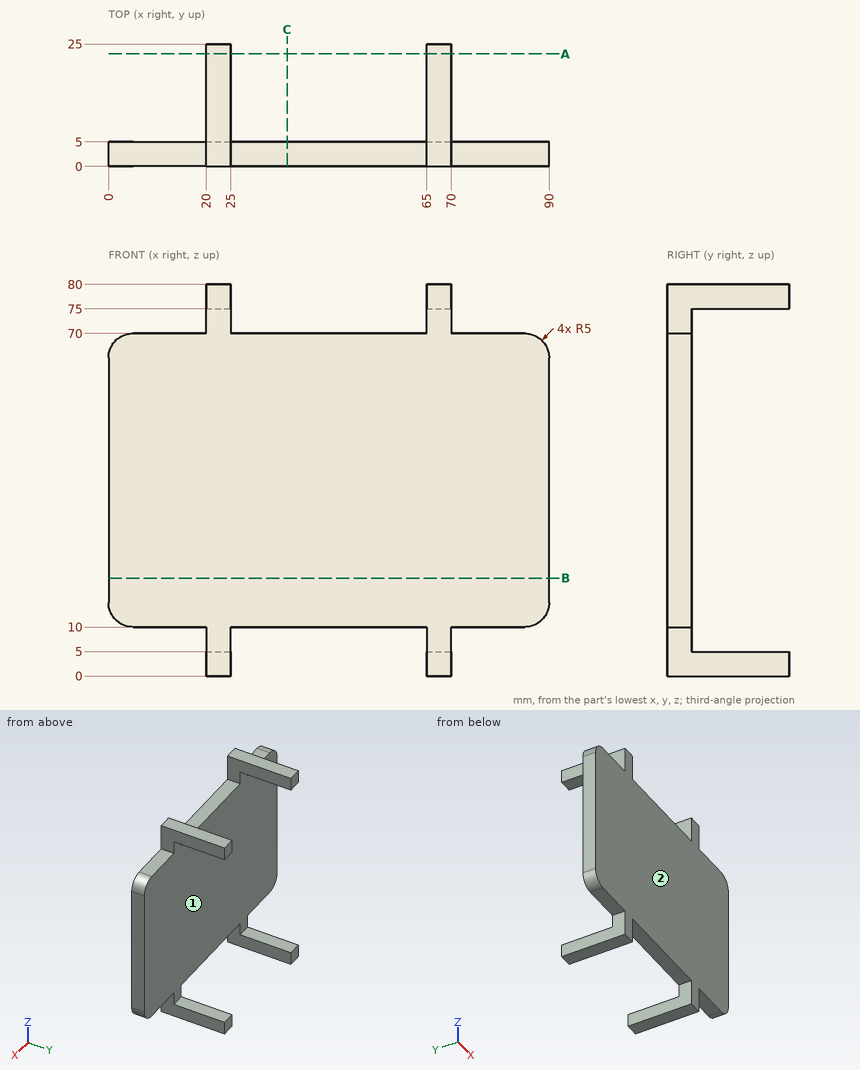
For this review, use the dimensioned drawing (mm, ordinates from the lowest corner) and the shaded views. A direction names the side the tool comes from. Round coordinates to 2 decimals unless told otherwise and drop trailing zeros. Write each loop counter-clockwise with the first axis right and the second up, starting at its lowest first coordinate (ties: lowest second). Pieces come first, ordered by that corner, then holes. Notation, with made-up numbers: (85.25, 16.5) - (103.25, 16.5) arc R30 ccw to (103.25, 45.5) - close; hole circle Ø2 at (58.25, -8.75). An arc over 180 degrees is marked (long way). Answer as CSV lines item,"result". Start each with the question number.
(1) For the marked faces 1 and 2, list the 3-axis set-ups (+Z, -Z, +X, -X, +Y, -Y) from which the entire face can be reached by the end or side of a thin tool; tool diameter is ignored.
(2) For pin 1 Ø8 at (y, z) = (7, 3.5) entering from -X; pin 2 Ø3 at (y, z) = (17.5, 76) entering from +X; pin 3 Ø1.5 at (x, y) = (15.5, 3) entering from +Z, all flat-tipped, find the tip position at first contact; note any pin that passes through.
(3) To check wall thickness, follow line 1 (Z direction, x = 68.5, y = 20.75); line 2 (X direction, y = 4, z = 74); line 3 (Y direction, x = 27, z = 50). State the ranges of each line that lie inside material, in increasing order.
(4) We need section C-C on x = 36.5. State the section outline as (y, z) points.
(5) We need section B-B on z = 20. State the section outline as (x, y) points, plus the area to 3 significant figures.
(6) We need section A-A on y = 23. State the section outline as (x, z) points, plus the area to 3 significant figures.
Worked answers:
1,face 1,"+X, -X, +Y"
1,face 2,"+Z, -Z, +X, -X, -Y"
2,pin 1,"x = 20"
2,pin 2,"x = 70"
2,pin 3,"z = 70"
3,line 1,"0 to 5, 75 to 80"
3,line 2,"20 to 25, 65 to 70"
3,line 3,"0 to 5"
4,outline,"(0, 10) - (5, 10) - (5, 70) - (0, 70) - close"
5,outline,"(0, 0) - (90, 0) - (90, 5) - (0, 5) - close"
5,area,"450 mm²"
6,outline,"(20, 0) - (25, 0) - (25, 5) - (20, 5) - close; (20, 75) - (25, 75) - (25, 80) - (20, 80) - close; (65, 0) - (70, 0) - (70, 5) - (65, 5) - close; (65, 75) - (70, 75) - (70, 80) - (65, 80) - close"
6,area,"100 mm²"
